Geometry check sheet. Reference: drawing and pictorial views, mm from the part's lowest x, y, z. Round coordinates to 2 decimals unless told otherwise and drop trailing zeros. Write each loop counter-clockwise with the first axis right and the second up, starting at its lowest first coordinate (ties: lowest second). Pieces come first, ordered by that corner, then holes. Notation, with made-up numbers: M -12,12.25 L 14,12.25 A15 cw 14,30.25 Z; hole C 85.25,82 d9. An arc over 180 degrees is marked long. One line per question, with ' | ' between items.
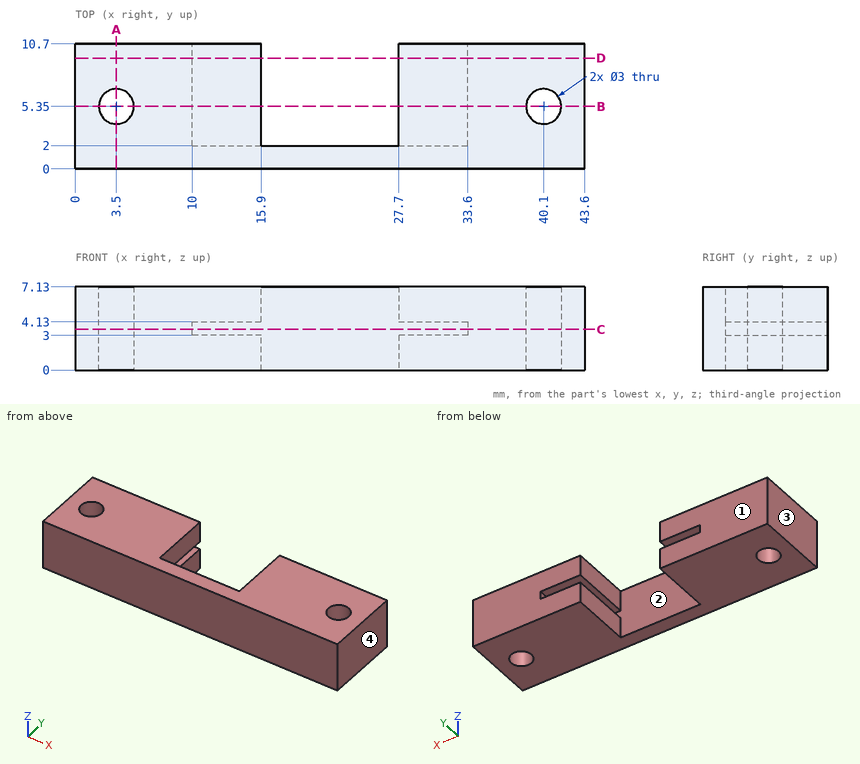
1. Section check C-C, the plane z = 3.5. Record the cut outline in (x, y).
Results:
outline: M 0,0 L 43.6,0 L 43.6,10.7 L 33.6,10.7 L 33.6,2 L 10,2 L 10,10.7 L 0,10.7 Z; hole C 3.5,5.35 d3; hole C 40.1,5.35 d3
2. Section check A-A, the plane x = 3.5. Record the cut outline in (y, z).
Results:
outline: M 0,0 L 3.85,0 L 3.85,7.13 L 0,7.13 Z; M 6.85,0 L 10.7,0 L 10.7,7.13 L 6.85,7.13 Z
3. Go/stop test with flat-tipped pins: P1, Ø1.2, axis at y = 6, z = 3.5, coming from the -X side; P2, Ø2, axis at x = 20.5, z = 3.5, coming from the +Y side; P3, Ø2.5, axis at x = 3.5, y = 5.35, coming from the -Z side. Record where each tip stops, or that it passes through.
Results:
P1: stops at x = 0 | P2: stops at y = 2 | P3: passes through
4. Section check B-B, the plane y = 5.35. Record the cut outline in (x, z), then the cut area to 3 significant figures.
Results:
outline: M 0,0 L 2,0 L 2,7.13 L 0,7.13 Z; M 5,0 L 15.9,0 L 15.9,3 L 10,3 L 10,4.13 L 15.9,4.13 L 15.9,7.13 L 5,7.13 Z; M 27.7,0 L 38.6,0 L 38.6,7.13 L 27.7,7.13 L 27.7,4.13 L 33.6,4.13 L 33.6,3 L 27.7,3 Z; M 41.6,0 L 43.6,0 L 43.6,7.13 L 41.6,7.13 Z | area: 171 mm2
5. Thickness scan on line 1 (Y direction, x = 40.1, z = 5.25); line 2 (Z direction, x = 30, y = 7.25); line 3 (X direction, y = 7, z = 6). Record the ranges inside material, lowest first.
Results:
line 1: y = 0 to 3.85, 6.85 to 10.7 | line 2: z = 0 to 3, 4.13 to 7.13 | line 3: x = 0 to 15.9, 27.7 to 43.6
6. Mould release check, pull along X, two halves, no side actions. Record for the marked faces 1, 2, 3 and 4: pulls with the +X half, pulls with the -X half, needs draft (parallel to the pull), parting line crosses it, or undercut.
Results:
face 1: needs draft | face 2: undercut | face 3: pulls with the -X half | face 4: pulls with the +X half
7. Section check D-D, the plane y = 9.5. Record the cut outline in (x, z).
Results:
outline: M 0,0 L 15.9,0 L 15.9,3 L 10,3 L 10,4.13 L 15.9,4.13 L 15.9,7.13 L 0,7.13 Z; M 27.7,0 L 43.6,0 L 43.6,7.13 L 27.7,7.13 L 27.7,4.13 L 33.6,4.13 L 33.6,3 L 27.7,3 Z
